The drawing under review shows one solid part. Ordinate dimensions are in mm from its lowest x, y, z. Round coordinates to 2 decimals unless told otherwise and drop trailing zeros. Order: outer loops, then holes, each group sorted by start corner. A loop starts at its lowest first (then second) coordinate and runs counter-clockwise, first axis right, second up. Notation, with made-up numbers: M 51.5,-23 L 101.5,-23 A22 ccw 101.5,14 Z; hole C 60.25,76 d5. An arc over 180 degrees is marked long. Answer as a JSON object with one key per item and string values. Group by question number.
1) Insertion check: pin 1 Ø3 at (x, z) = (4, 2.5) entering from +Y (1 decimal). The pin has a flat end and moves straight along its axis. Give the tip position at first contact, or say it passes through.
2) To check wall thickness, follow line 1 (Y direction, x = 2.5, z = 0.75) (1 decimal); line 2 (X direction, y = 6, z = 1.5); line 3 (Y direction, x = 7.5, z = 3.25) (1 decimal). State the ranges of each line that lie inside material, in increasing order.
3) The part is to be moulded in two halves that separate along Y. For the marked faces 1, 2 and 3, say which applies: +Y half, -Y half, draft (parallel to the pull), parting line (faces both ways), or undercut.
4) Consider section C-C, the plane y = 13. Write out the cut boundary in (x, z).
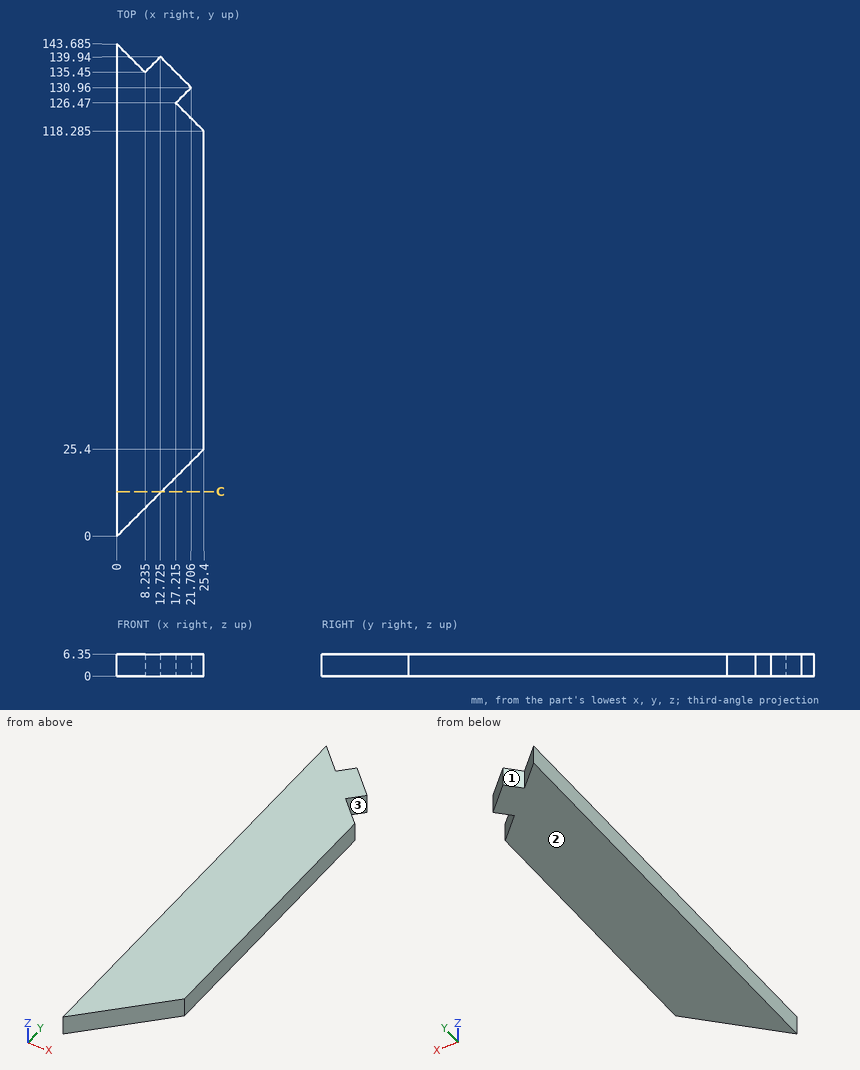
Results list:
{
 "1": {"pin 1": "y = 141.2"},
 "2": {"line 1": "2.5 to 141.2", "line 2": "0 to 6", "line 3": "7.5 to 136.2"},
 "3": {"face 1": "+Y half", "face 2": "draft", "face 3": "undercut"},
 "4": {"outline": "M 0,0 L 13,0 L 13,6.35 L 0,6.35 Z"}
}
